The listing builds one solid part. Answer for the finished solid, in the listing's coordinates (mm). A direction names the side the tool comes from. Give positions to 0.01 mm unless a question says otherwise; leave off trailing zeros. Loops run counter-clockwise (first coordinate to the right, second up) from the corner with the lowest first, then second, coordinate; pieces in that order, holes last. Notation, with made-up numbers: M 8.25,-16.5 L 66.25,-16.5 A26 ccw 66.25,18.5 Z; hole C 33,14 d10. An arc over 180 degrees is marked long. Use one line per item in the form item = value. Start each with the question number.
1. The part is cut by section C-C (z = 11.5). Write down the section's boundary in (x, y).
2. The part is cut by section B-B (x = 9.6). Write down the section's boundary in (y, z).
3. The part is cut by section A-A (y = 98.3). Write down the section's boundary in (x, z).
4. Each of these flat-tipped pins is pushed along its axis until it touches: pin 1 Ø3 at (x, y) = (8.5, 97) entering from +Z; pin 2 Ø1.5 at (x, z) = (10, 16) entering from +Y; pin 3 Ø1 at (y, z) = (100, 14.5) entering from -X. Where does it stop, or does it pass through?
5. Straight lines are drawn through the part: line 1 (Z direction, x = 9.75, y = 95.9); line 2 (X direction, y = 98.3, z = 13); line 3 (Y direction, x = 9.55, z = 16.25). For each, find the intervals that lie inside material, in ascending order. Write a range as from..to.
6. For faces 1 (the face through (9, 101, 11.1)), 2 (the face through (10, 98, 19.1)), determine the directions among +Z, -Z, +X, -X, +Y, -Y from which every point of the face is accessible in a straight line to the end or side of a thin tool.
7. The part is cut by section D-D (x = 11.9). Write down the section's boundary in (y, z).
from build123d import *

# Parameters (mm, degrees)
CYLINDER019_R     = 2.2
CYLINDER019_DEPTH = 9
CYLINDER021_R     = 3
CYLINDER021_DEPTH = 1
FILLET_R          = 1


with BuildPart() as obj1_c:
    # Cylinder019 → Cylinder019 (new body)
    with BuildSketch(Plane(origin=(9.6, 98.3, 10.1), x_dir=(1, 0, 0), z_dir=(0, 0, 1))):
        Circle(CYLINDER019_R)
    extrude(amount=CYLINDER019_DEPTH)


with BuildPart() as obj1:
    # Cylinder021 → Cylinder021 (new body)
    with BuildSketch(Plane(origin=(9.6, 98.3, 10.1), x_dir=(1, 0, 0), z_dir=(0, 0, 1))):
        Circle(CYLINDER021_R)
    extrude(amount=CYLINDER021_DEPTH)

    # Fusion032: union obj1_c
    add(obj1_c.part)

    # Fillet
    fillet_edges = [obj1.edges().sort_by_distance(p)[0] for p in [
        (7.4, 98.3, 19.1),
    ]]
    fillet(fillet_edges, radius=FILLET_R)


solid = obj1.part
Derived:
q1.outline = C 9.6,98.3 d4.4
q2.outline = M 95.3,10.1 L 101.3,10.1 L 101.3,11.1 L 100.5,11.1 L 100.5,18.1 A1 ccw 99.5,19.1 L 97.1,19.1 A1 ccw 96.1,18.1 L 96.1,11.1 L 95.3,11.1 Z
q3.outline = M 6.6,10.1 L 12.6,10.1 L 12.6,11.1 L 11.8,11.1 L 11.8,18.1 A1 ccw 10.8,19.1 L 8.4,19.1 A1 ccw 7.4,18.1 L 7.4,11.1 L 6.6,11.1 Z
q4.pin_1 = 19.1
q4.pin_2 = 100.5
q4.pin_3 = 7.76
q5.line_1 = 10.1..11.1
q5.line_2 = 7.4..11.8
q5.line_3 = 96.1..100.5
q6.face_1 = +Z
q6.face_2 = +Z, +X, -X, +Y, -Y
q7.outline = M 96.37,10.1 L 100.23,10.1 L 100.23,11.1 L 96.37,11.1 Z
